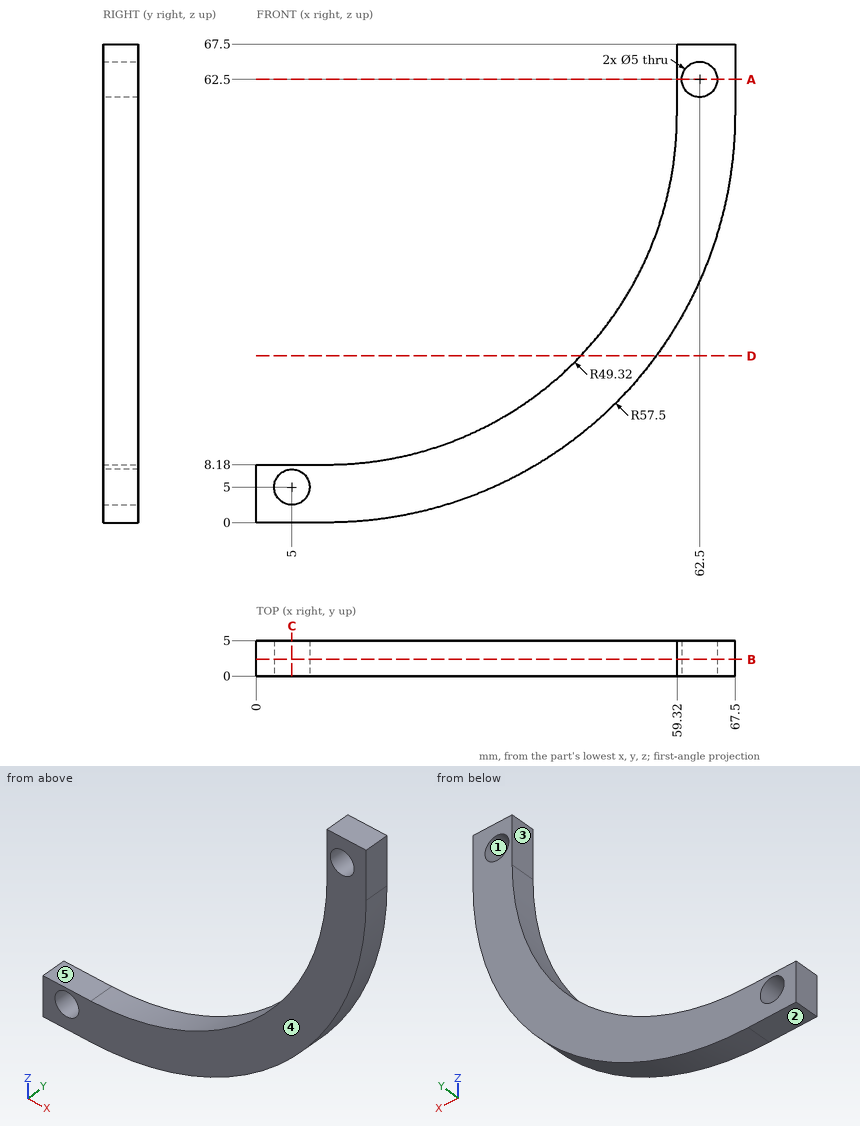
Job drawing, mm, ordinate dimensions from the low corner. One solid piece. A direction names the side the tool comes from. Coordinates: 2 decimals unless noted, no trailing zeros. Order: outer loops, then holes, each group sorted by start corner. A loop starts at its lowest first (then second) coordinate and runs counter-clockwise, first axis right, second up. Notation, with made-up numbers: M 27.25,49.25 L 43.25,49.25 A31 ccw 43.25,75.25 Z; hole C -26.75,87.5 d7. An arc over 180 degrees is marked long. Return JSON: item names as keys, results as strings.
1. Tool access for the marked faces 4 and 5: list every direction of +Z, -Z, +X, -X, +Y, -Y with a clear straight run to the whole face (end or side of a thin tool).
Ans:
{"face 4": "+Z, -Z, +X, -X, -Y", "face 5": "+Z, -X, +Y, -Y"}
2. Saw through at B-B (y = 2.35). Give the cut face in (x, z), and give its area (3 significant figures).
Ans:
{"outline": "M 0,0 L 10,0 A57.5 ccw 67.5,57.5 L 67.5,67.5 L 59.32,67.5 L 59.32,57.5 A49.32 cw 10,8.18 L 0,8.18 Z; hole C 5,5 d5; hole C 62.5,62.5 d5", "area": "811 mm^2"}
3. Saw through at D-D (z = 23.5). Give the cut face in (x, y), and give its area (3 significant figures).
Ans:
{"outline": "M 45.73,0 L 56.37,0 L 56.37,5 L 45.73,5 Z", "area": "53.2 mm^2"}
4. Drill centre lines: probe 1 along X at (y, z) = (1.5, 58); probe 2 along X at (y, z) = (3, 5); probe 3 along Z at (x, y) = (10.5, 3.75). Where is each one in solid material? Low to high.
Ans:
{"probe 1": "59.32 to 67.5", "probe 2": "0 to 2.5, 7.5 to 33.45", "probe 3": "0 to 8.18"}
5. Saw through at A-A (z = 62.5). Give the cut face in (x, y).
Ans:
{"outline": "M 59.32,0 L 60,0 L 60,5 L 59.32,5 Z; M 65,0 L 67.5,0 L 67.5,5 L 65,5 Z"}
6. Flat gauge pins, fed straight in: pin 1 (1.5 mm diameter, centred on y = 1.5, z = 63, fed in from -X); pin 2 (1.5 mm diameter, centred on x = 56.5, y = 4, fed in from -Z); pin 3 (1.5 mm diameter, centred on x = 53, y = 2.5, fed in from -Z). Where does each tip first touch, or does it go through?
Ans:
{"pin 1": "x = 59.32", "pin 2": "z = 22.67", "pin 3": "z = 18.5"}
7. Pull direction Z, two halves, no side cores. Call the marked faces 1, 2 and 3: +Z half, -Z half, draft (parallel to the pull), parting line (faces both ways), or undercut.
Ans:
{"face 1": "undercut", "face 2": "-Z half", "face 3": "draft"}
8. Saw through at C-C (x = 5). Give the cut face in (y, z).
Ans:
{"outline": "M 0,0 L 5,0 L 5,2.5 L 0,2.5 Z; M 0,7.5 L 5,7.5 L 5,8.18 L 0,8.18 Z"}
